```python
from build123d import *

# Parameters (mm, degrees)
BOX019_W               = 20
BOX019_H               = 30
BOX019_DEPTH           = 15
BOX018_W               = 24
BOX018_H               = 34
BOX018_DEPTH           = 15
CYLINDER011_R          = 1.6
CYLINDER011_DEPTH      = 30
BOX013_W               = 6.5
BOX013_H               = 5
BOX013_DEPTH           = 2.5
BOX014_W               = 8
BOX014_H               = 6
BOX014_DEPTH           = 10
CUT006_PLACEMENT_ANGLE = 180
CYLINDER010_R          = 1.6
CYLINDER010_DEPTH      = 30
BOX012_W               = 6.5
BOX012_H               = 5
BOX012_DEPTH           = 2.5
BOX011_W               = 8
BOX011_H               = 6
BOX011_DEPTH           = 10
CYLINDER009_R          = 1.6
CYLINDER009_DEPTH      = 30
BOX010_W               = 6.5
BOX010_H               = 5
BOX010_DEPTH           = 2.5
BOX009_W               = 8
BOX009_H               = 6
BOX009_DEPTH           = 10
BOX004_W               = 3
BOX004_H               = 80
BOX004_DEPTH           = 30
BOX003_W               = 3
BOX003_H               = 80
BOX003_DEPTH           = 30
BOX001_W               = 65
BOX001_H               = 3
BOX001_DEPTH           = 30
CYLINDER001_R          = 1.5
CYLINDER001_DEPTH      = 10
CYLINDER002_R          = 1.5
CYLINDER002_DEPTH      = 10
CYLINDER003_R          = 1.5
CYLINDER003_DEPTH      = 10
BOX_W                  = 65
BOX_H                  = 78
BOX_DEPTH              = 3
CYLINDER_R             = 1.5
CYLINDER_DEPTH         = 10
BOX008_W               = 10
BOX008_H               = 10
BOX008_DEPTH           = 3
BOX007_W               = 8
BOX007_H               = 10
BOX007_DEPTH           = 3
CYLINDER008_R          = 7
CYLINDER008_DEPTH      = 10
BOX002_W               = 65
BOX002_H               = 3
BOX002_DEPTH           = 30
CYLINDER012_R          = 1.6
CYLINDER012_DEPTH      = 30
BOX015_W               = 6.5
BOX015_H               = 5
BOX015_DEPTH           = 2.5
BOX016_W               = 8
BOX016_H               = 6
BOX016_DEPTH           = 10
CUT007_PLACEMENT_ANGLE = 180


with BuildPart() as cube015:
    # Box019 → Box019 (new body)
    with BuildSketch(Plane(origin=(-17, 70, 2), x_dir=(1, 0, 0), z_dir=(0, 0, 1))):
        with Locations((10, 15)):
            Rectangle(BOX019_W, BOX019_H)
    extrude(amount=BOX019_DEPTH)


with BuildPart() as cut009:
    # Box018 → Box018 (new body)
    with BuildSketch(Plane(origin=(-19, 68, 0), x_dir=(1, 0, 0), z_dir=(0, 0, 1))):
        with Locations((12, 17)):
            Rectangle(BOX018_W, BOX018_H)
    extrude(amount=BOX018_DEPTH)

    # Cut009: cut Cube015
    add(cube015.part, mode=Mode.SUBTRACT)


with BuildPart() as cylinder011:
    # Cylinder011 → Cylinder011 (new body)
    with BuildSketch(Plane(origin=(6, 29, 0), x_dir=(1, 0, 0), z_dir=(0, 0, 1))):
        Circle(CYLINDER011_R)
    extrude(amount=CYLINDER011_DEPTH)


with BuildPart() as cube009:
    # Box013 → Box013 (new body)
    with BuildSketch(Plane(origin=(3, 27, 20), x_dir=(1, 0, 0), z_dir=(0, 0, 1))):
        with Locations((3.25, 2.5)):
            Rectangle(BOX013_W, BOX013_H)
    extrude(amount=BOX013_DEPTH)


with BuildPart() as cut006:
    # Box014 → Box014 (new body)
    with BuildSketch(Plane(origin=(2.5, 25.5, 15), x_dir=(1, 0, 0), z_dir=(0, 0, 1))):
        with Locations((4, 3)):
            Rectangle(BOX014_W, BOX014_H)
    extrude(amount=BOX014_DEPTH)

    # Cut005: cut Cube009
    add(cube009.part, mode=Mode.SUBTRACT)

    # Cut006: cut Cylinder011
    add(cylinder011.part, mode=Mode.SUBTRACT)


with BuildPart() as cut006_1:
    # Cut006 placement: moved
    add(cut006.part.moved(Location((69, 125, 5))).rotate(Axis((69, 125, 5), (0, 0, 1)), CUT006_PLACEMENT_ANGLE))


with BuildPart() as cylinder010:
    # Cylinder010 → Cylinder010 (new body)
    with BuildSketch(Plane(origin=(6, 29, 0), x_dir=(1, 0, 0), z_dir=(0, 0, 1))):
        Circle(CYLINDER010_R)
    extrude(amount=CYLINDER010_DEPTH)


with BuildPart() as cube008:
    # Box012 → Box012 (new body)
    with BuildSketch(Plane(origin=(3, 27, 20), x_dir=(1, 0, 0), z_dir=(0, 0, 1))):
        with Locations((3.25, 2.5)):
            Rectangle(BOX012_W, BOX012_H)
    extrude(amount=BOX012_DEPTH)


with BuildPart() as cut003:
    # Box011 → Box011 (new body)
    with BuildSketch(Plane(origin=(2.5, 25.5, 15), x_dir=(1, 0, 0), z_dir=(0, 0, 1))):
        with Locations((4, 3)):
            Rectangle(BOX011_W, BOX011_H)
    extrude(amount=BOX011_DEPTH)

    # Cut004: cut Cube008
    add(cube008.part, mode=Mode.SUBTRACT)

    # Cut003: cut Cylinder010
    add(cylinder010.part, mode=Mode.SUBTRACT)


with BuildPart() as cut003_1:
    # Cut003 placement: moved
    add(cut003.part.moved(Location((56, -1, 5))))


with BuildPart() as cylinder:
    # Cylinder009 → Cylinder009 (new body)
    with BuildSketch(Plane(origin=(6, 29, 0), x_dir=(1, 0, 0), z_dir=(0, 0, 1))):
        Circle(CYLINDER009_R)
    extrude(amount=CYLINDER009_DEPTH)


with BuildPart() as cube006:
    # Box010 → Box010 (new body)
    with BuildSketch(Plane(origin=(3, 27, 20), x_dir=(1, 0, 0), z_dir=(0, 0, 1))):
        with Locations((3.25, 2.5)):
            Rectangle(BOX010_W, BOX010_H)
    extrude(amount=BOX010_DEPTH)


with BuildPart() as cut002:
    # Box009 → Box009 (new body)
    with BuildSketch(Plane(origin=(2.5, 25.5, 15), x_dir=(1, 0, 0), z_dir=(0, 0, 1))):
        with Locations((4, 3)):
            Rectangle(BOX009_W, BOX009_H)
    extrude(amount=BOX009_DEPTH)

    # Cut001: cut Cube006
    add(cube006.part, mode=Mode.SUBTRACT)

    # Cut002: cut Cylinder
    add(cylinder.part, mode=Mode.SUBTRACT)


with BuildPart() as cut002_1:
    # Cut002 placement: moved
    add(cut002.part.moved(Location((0, -1, 5))))


with BuildPart() as cube004:
    # Box004 → Box004 (new body)
    with BuildSketch(Plane(origin=(65, 22, 0), x_dir=(1, 0, 0), z_dir=(0, 0, 1))):
        with Locations((1.5, 40)):
            Rectangle(BOX004_W, BOX004_H)
    extrude(amount=BOX004_DEPTH)


with BuildPart() as cube003:
    # Box003 → Box003 (new body)
    with BuildSketch(Plane(origin=(0, 22, 0), x_dir=(1, 0, 0), z_dir=(0, 0, 1))):
        with Locations((1.5, 40)):
            Rectangle(BOX003_W, BOX003_H)
    extrude(amount=BOX003_DEPTH)


with BuildPart() as cube001:
    # Box001 → Box001 (new body)
    with BuildSketch(Plane(origin=(0, 22, 0), x_dir=(1, 0, 0), z_dir=(0, 0, 1))):
        with Locations((32.5, 1.5)):
            Rectangle(BOX001_W, BOX001_H)
    extrude(amount=BOX001_DEPTH)


with BuildPart() as cilindro001:
    # Cylinder001 → Cylinder001 (new body)
    with BuildSketch(Plane(origin=(42, 43, 0), x_dir=(1, 0, 0), z_dir=(0, 0, 1))):
        Circle(CYLINDER001_R)
    extrude(amount=CYLINDER001_DEPTH)


with BuildPart() as cilindro002:
    # Cylinder002 → Cylinder002 (new body)
    with BuildSketch(Plane(origin=(57.5, 94, 0), x_dir=(1, 0, 0), z_dir=(0, 0, 1))):
        Circle(CYLINDER002_R)
    extrude(amount=CYLINDER002_DEPTH)


with BuildPart() as cilindro003:
    # Cylinder003 → Cylinder003 (new body)
    with BuildSketch(Plane(origin=(9, 95, 0), x_dir=(1, 0, 0), z_dir=(0, 0, 1))):
        Circle(CYLINDER003_R)
    extrude(amount=CYLINDER003_DEPTH)


with BuildPart() as cube:
    # Box → Box (new body)
    with BuildSketch(Plane(origin=(0, 22, 0), x_dir=(1, 0, 0), z_dir=(0, 0, 1))):
        with Locations((32.5, 39)):
            Rectangle(BOX_W, BOX_H)
    extrude(amount=BOX_DEPTH)


with BuildPart() as fusion:
    # Cylinder → Cylinder (new body)
    with BuildSketch(Plane(origin=(14, 43, 0), x_dir=(1, 0, 0), z_dir=(0, 0, 1))):
        Circle(CYLINDER_R)
    extrude(amount=CYLINDER_DEPTH)

    # Fusion: union Cilindro001, Cilindro002, Cilindro003, Cube
    add(cilindro001.part)
    add(cilindro002.part)
    add(cilindro003.part)
    add(cube.part)


with BuildPart() as cubo008:
    # Box008 → Box008 (new body)
    with BuildSketch(Plane(origin=(28, 96, 20), x_dir=(1, 0, 0), z_dir=(0, 0, 1))):
        with Locations((5, 5)):
            Rectangle(BOX008_W, BOX008_H)
    extrude(amount=BOX008_DEPTH)


with BuildPart() as fusion001006:
    # Box007 → Box007 (new body)
    with BuildSketch(Plane(origin=(29, 96, 18), x_dir=(1, 0, 0), z_dir=(0, 0, 1))):
        with Locations((4, 5)):
            Rectangle(BOX007_W, BOX007_H)
    extrude(amount=BOX007_DEPTH)

    # Fusion001006: union Cubo008
    add(cubo008.part)


with BuildPart() as fusion001006_1:
    # Fusion001006 placement: moved
    add(fusion001006.part.moved(Location((0, 0, 1))))


with BuildPart() as fusion001005:
    # Cylinder008 → Cylinder008 (new body)
    with BuildSketch(Plane(origin=(17, 106, 12), x_dir=(1, 0, 0), z_dir=(0, -1, 0))):
        Circle(CYLINDER008_R)
    extrude(amount=CYLINDER008_DEPTH)

    # Fusion001005: union Fusion001006
    add(fusion001006_1.part)


with BuildPart() as fusion001005_1:
    # Fusion001005 placement: moved
    add(fusion001005.part.moved(Location((0, 1, -0.5))))


with BuildPart() as caja:
    # Box002 → Box002 (new body)
    with BuildSketch(Plane(origin=(0, 99, 0), x_dir=(1, 0, 0), z_dir=(0, 0, 1))):
        with Locations((32.5, 1.5)):
            Rectangle(BOX002_W, BOX002_H)
    extrude(amount=BOX002_DEPTH)

    # Cut: cut Fusion001005
    add(fusion001005_1.part, mode=Mode.SUBTRACT)

    # Fusion001007: union Cube004, Cube003, Cube001, Fusion
    add(cube004.part)
    add(cube003.part)
    add(cube001.part)
    add(fusion.part)


with BuildPart() as cylinder012:
    # Cylinder012 → Cylinder012 (new body)
    with BuildSketch(Plane(origin=(6, 29, 0), x_dir=(1, 0, 0), z_dir=(0, 0, 1))):
        Circle(CYLINDER012_R)
    extrude(amount=CYLINDER012_DEPTH)


with BuildPart() as cube011:
    # Box015 → Box015 (new body)
    with BuildSketch(Plane(origin=(3, 27, 20), x_dir=(1, 0, 0), z_dir=(0, 0, 1))):
        with Locations((3.25, 2.5)):
            Rectangle(BOX015_W, BOX015_H)
    extrude(amount=BOX015_DEPTH)


with BuildPart() as fusion001009:
    # Box016 → Box016 (new body)
    with BuildSketch(Plane(origin=(2.5, 25.5, 15), x_dir=(1, 0, 0), z_dir=(0, 0, 1))):
        with Locations((4, 3)):
            Rectangle(BOX016_W, BOX016_H)
    extrude(amount=BOX016_DEPTH)

    # Cut008: cut Cube011
    add(cube011.part, mode=Mode.SUBTRACT)

    # Cut007: cut Cylinder012
    add(cylinder012.part, mode=Mode.SUBTRACT)


with BuildPart() as fusion001009_1:
    # Cut007 placement: moved
    add(fusion001009.part.moved(Location((12, 125, 5))).rotate(Axis((12, 125, 5), (0, 0, 1)), CUT007_PLACEMENT_ANGLE))

    # Fusion001008: union Cut006, Cut003, Cut002, caja
    add(cut006_1.part)
    add(cut003_1.part)
    add(cut002_1.part)
    add(caja.part)

    # Fusion001009: union Cut009
    add(cut009.part)


solid = fusion001009_1.part
```
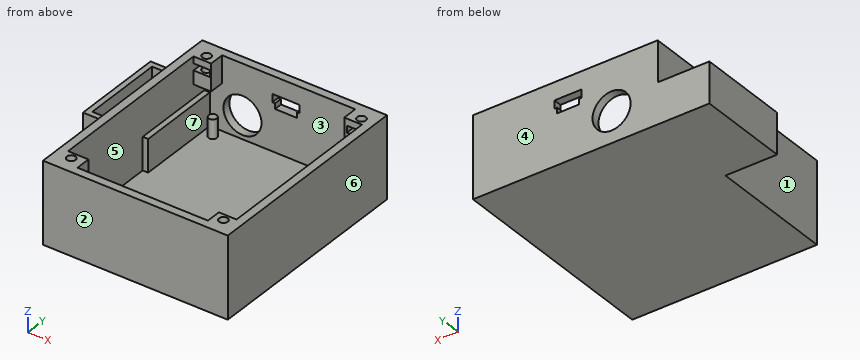
Could you check a few things on this model? Use its own coordinates, in mm. Face numbers are marked on the shaded views. A direction names the side the tool comes from. Give positions to 0.01 mm unless a question says otherwise; leave off trailing zeros. Write each loop counter-clockwise with the first axis right and the second up, starting at its lowest first coordinate (ties: lowest second). Pieces come first, ordered by that corner, then holes. Notation, with made-up numbers: (-31.5, 58.25) -> (3.5, 58.25) arc R18 ccw to (3.5, 92.25) -> close; hole circle Ø2 at (17, 61.5). An arc over 180 degrees is marked (long way). Write each question's results on one line, items separated by ' | '.
1. I want a section at B-B, the plane z = 11.5. Write out the boundary of the cut face in (x, y).
Check sheet entries:
outline: (-19, 68) -> (0, 68) -> (0, 22) -> (68, 22) -> (68, 102) -> (24, 102) -> (24, 99) -> (65, 99) -> (65, 25) -> (3, 25) -> (3, 68) -> (5, 68) -> (5, 99) -> (10, 99) -> (10, 102) -> (-19, 102) -> close; hole (-17, 70) -> (0, 70) -> (0, 100) -> (-17, 100) -> close
2. Will these pins go through, and if not, where does the flat tip stop? pin 1 Ø1.5 at (x, y) = (15.5, 76.5) entering from +Z; pin 2 Ø2 at (y, z) = (28, 26) entering from -X.
Check sheet entries:
pin 1: stops at z = 3 | pin 2: stops at x = 0
3. I need wall thicknesses on L1, parallel to X at y = 81, z = 5.25; L2, parallel to Y at x = 6, z = 23.1; L3, parallel to X at y = 95, z = 25.5. Which ranges of each line are inside material? Lowest first, please.
Check sheet entries:
L1: x = -19 to -17, 0 to 5, 65 to 68 | L2: y = 22 to 26.4, 29.6 to 30.5, 93.5 to 94.4, 97.6 to 102 | L3: x = 0 to 3, 9 to 9.5, 58.5 to 59.5, 65 to 68
4. I want a section at A-A, the plane x = 30. Write out the boundary of the cut face in (y, z).
Check sheet entries:
outline: (22, 0) -> (102, 0) -> (102, 18.5) -> (99, 18.5) -> (99, 3) -> (25, 3) -> (25, 30) -> (22, 30) -> close; (99, 23.5) -> (102, 23.5) -> (102, 30) -> (99, 30) -> close
5. On a 3-axis mill with a long thin cutter (end or side, diameter ignored), from which of +Z, -Z, +X, -X, +Y, -Y can I reach the whole of each face in a straight line? I mean the marked faces 1, 2 and 3. Say none if no direction works.
Check sheet entries:
face 1: +Z | face 2: +Z, -Z, +X, -X, -Y | face 3: none
6. I want a section at C-C, the plane x = 54.5. Write out the boundary of the cut face in (y, z).
Check sheet entries:
outline: (22, 0) -> (102, 0) -> (102, 30) -> (99, 30) -> (99, 3) -> (25, 3) -> (25, 30) -> (22, 30) -> close
7. If we mould it in two halves opening along Y, with no side actions, what happens to the marked faces 4, 5, 6 and 7? For each: released by +Y, released by -Y, zero draft, split by the parting line, or undercut.
Check sheet entries:
face 4: released by +Y | face 5: undercut | face 6: zero draft | face 7: undercut
8. I want a section at D-D, the plane y = 28. Count the separate pieces of the cut face and the enclosed holes in it, then the cut area to 3 significant figures.
Check sheet entries:
separate pieces: 3 | enclosed holes: 0 | area: 427 mm²
